Here's the drawing with two shaded views (mm, measured from the low corner). I have some questions. Round coordinates to 2 decimals unless told otherwise and drop trailing zeros. Order: outer loops, then holes, each group sorted by start corner. A loop starts at its lowest first (then second) coordinate and runs counter-clockwise, first axis right, second up.
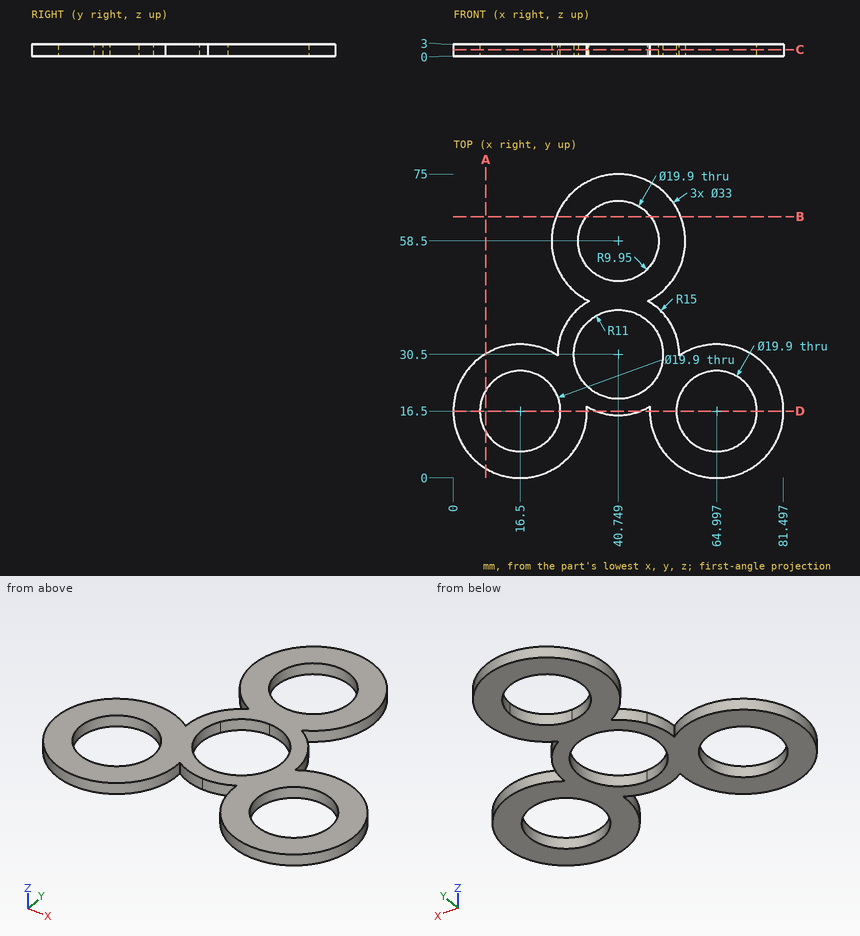
Q1. Imagine slicing it at A-A, the plane x = 8. Please give me the cut outline in (y, z).
Q2. For P1, Ø1.5, axis at y = 22, z = 2, coming from the +X side; P2, Ø5, axis at x = 13.5, y = 11, coming from the -Z side; P3, Ø1.5, axis at y = 51.5, z = 1, coming from the -X side, each with a flat end and sliding along its axis, tell me the tip position at first contact or that it passes through.
Q3. Imagine slicing it at C-C, the plane z = 1.6. State how many separate pieces and enclosed holes the cut face has, then the cut area to 3 significant figures.
Q4. I need wall thicknesses on L1, parallel to Y at x = 16.5, z = 0.9; L2, parallel to X at y = 14, z = 0.9; L3, parallel to X at y = 58.5, z = 0.6. Which ranges of each line are inside material? Lowest first, please.
Q5. Imagine slicing it at D-D, the plane y = 16.5. Please give me the cut outline in (x, z), then the cut area to 3 significant figures.
Q6. Imagine slicing it at B-B, the plane y = 64.5. Please give me the cut outline in (x, z), then the cut area to 3 significant figures.
Filled in:
1. outline: (2.36, 0) - (11.33, 0) - (11.33, 3) - (2.36, 3) - close; (21.67, 0) - (30.64, 0) - (30.64, 3) - (21.67, 3) - close
2. P1: stops at x = 80.8
2. P2: passes through
2. P3: stops at x = 25.48
3. separate pieces: 1
3. enclosed holes: 4
3. area: 1,860 mm2
4. L1: y = 0 to 6.55, 26.45 to 33
4. L2: x = 0.19 to 6.87, 26.13 to 32.81, 48.69 to 55.37, 74.63 to 81.31
4. L3: x = 24.25 to 30.8, 50.7 to 57.25
5. outline: (0, 0) - (6.55, 0) - (6.55, 3) - (0, 3) - close; (26.45, 0) - (33, 0) - (33, 3) - (26.45, 3) - close; (35.36, 0) - (46.13, 0) - (46.13, 3) - (35.36, 3) - close; (48.5, 0) - (55.05, 0) - (55.05, 3) - (48.5, 3) - close; (74.95, 0) - (81.5, 0) - (81.5, 3) - (74.95, 3) - close
5. area: 111 mm2
6. outline: (25.38, 0) - (32.81, 0) - (32.81, 3) - (25.38, 3) - close; (48.69, 0) - (56.12, 0) - (56.12, 3) - (48.69, 3) - close
6. area: 44.6 mm2
